The drawing under review shows one solid part. Ordinate dimensions are in mm from its lowest x, y, z. A direction names the side the tool comes from. Round coordinates to 2 decimals unless told otherwise and drop trailing zeros. Order: outer loops, then holes, each group sorted by start corner. A loop starts at its lowest first (then second) coordinate and runs counter-clockwise, first axis right, second up.
1) Clearance check with flat-ended pins moving along their axes: P1, Ø5, axis at x = 195, z = 86, coming from the +Y side; P2, Ø6, axis at x = 285.5, y = 190, coming from the +Z side; P3, Ø8, axis at x = 259.5, y = 120, coming from the -Z side. State where each tip first meets the part, or that it passes through.
2) To check wall thickness, follow L1, parallel to Y at x = 266, z = 100; L2, parallel to Y at x = 167.5, z = 159.5; L3, parallel to Z at x = 215, y = 95. State the ranges of each line that lie inside material, in increasing order.
3) Consider section D-D (z = 34). Give the boundary of the cut face in (x, y), then the cut area to 3 significant figures.
4) Consider section A-A (y = 200). Give the boundary of the cut face in (x, z).
5) Consider section C-C (z = 100). Give the boundary of the cut face in (x, y), then the cut area to 3 significant figures.
6) Consider section B-B (x = 273.5). Give the boundary of the cut face in (y, z), then the cut area to 3 significant figures.
7) Mouldability with a two-part tool opening along Y and no side actions: class the marked faces 4, 5, 6 and 7 as pulls with the +Y half, pulls with the -Y half, needs draft (parallel to the pull), parting line crosses it, or undercut.
8) Machinability: for the marked faces 1, 2 and 3, which of the approach directions +Z, -Z, +X, -X, +Y, -Y give a long, thin tool a straight path to every point of the face, cutting with its end or side? Answer none if there is none.
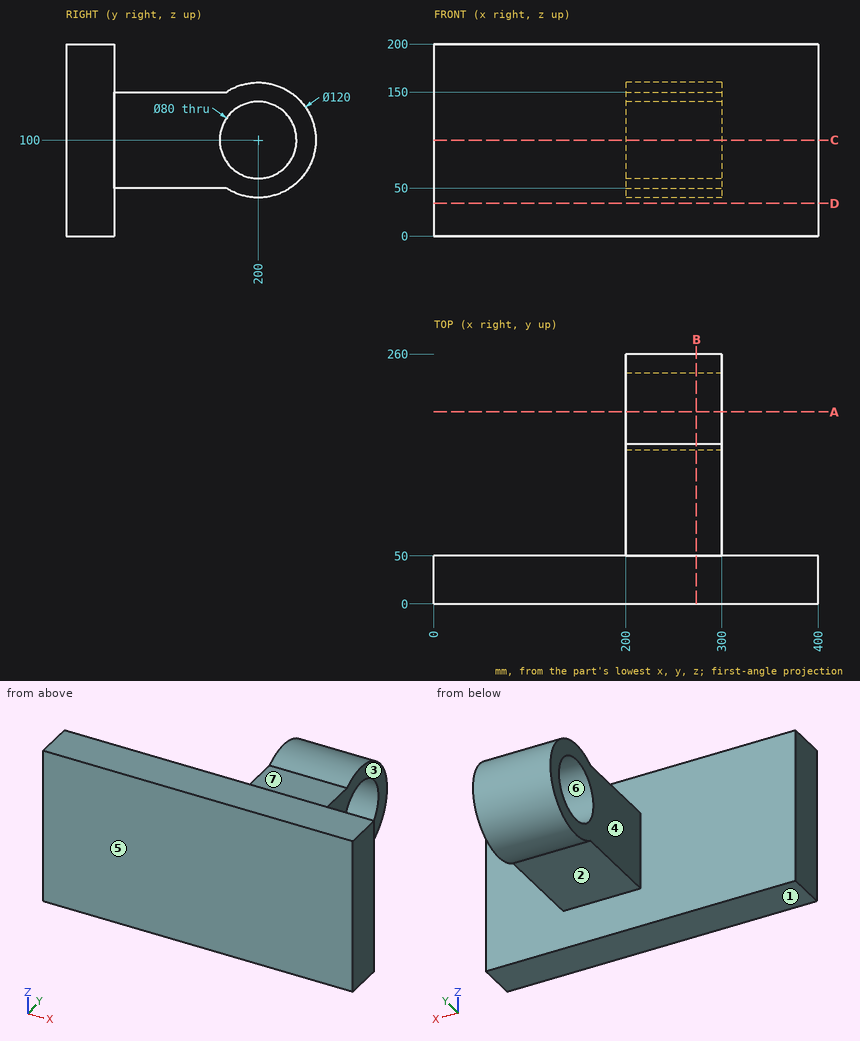
Answer below:
1. P1: stops at y = 50
1. P2: stops at z = 159.59
1. P3: stops at z = 50
2. L1: y = 0 to 160, 240 to 260
2. L2: y = 0 to 50
2. L3: z = 50 to 150
3. outline: (0, 0) - (400, 0) - (400, 50) - (0, 50) - close
3. area: 20,000 mm2
4. outline: (200, 40) - (300, 40) - (300, 60) - (200, 60) - close; (200, 140) - (300, 140) - (300, 160) - (200, 160) - close
5. outline: (0, 0) - (400, 0) - (400, 50) - (300, 50) - (300, 160) - (200, 160) - (200, 50) - (0, 50) - close; (200, 240) - (300, 240) - (300, 260) - (200, 260) - close
5. area: 33,000 mm2
6. outline: (0, 0) - (50, 0) - (50, 50) - (166.83, 50) arc R60 ccw (long way) to (166.83, 150) - (50, 150) - (50, 200) - (0, 200) - close; hole circle Ø80 at (200, 100)
6. area: 26,100 mm2
7. face 4: needs draft
7. face 5: pulls with the -Y half
7. face 6: undercut
7. face 7: undercut
8. face 1: -Z, +X, -X, +Y, -Y
8. face 2: -Z, +X, -X
8. face 3: +Z, -Z, +X, +Y
